For this review, take the finished solid that the model builds, in its own axes (mm). A direction names the side the tool comes from. Coordinates: 2 decimals unless noted, no trailing zeros. Write each loop counter-clockwise with the first axis right and the second up, starting at its lowest first coordinate (ties: lowest second). Pieces come first, ordered by that corner, then holes.
1) Insertion check: P1, Ø1.5, axis at x = 1, z = 23, coming from the -Y side; P2, Ø0.6, axis at x = 1.5, y = 0, coming from the -Z side. Each pin has a flat end and moves straight along its axis. Give the tip position at first contact, or say it passes through.
2) For faces 1 (the face through (0, 0, 26.6)), 2 (the face through (1, 0, -4)), list the 3-axis set-ups (+Z, -Z, +X, -X, +Y, -Y) from which the entire face can be reached by the end or side of a thin tool; tool diameter is ignored.
3) We need section A-A on z = -3. Write out the cut boundary in (x, y), then the cut area to 3 significant figures.
4) We need section B-B on z = 23.5. Write out the cut boundary in (x, y), then the cut area to 3 significant figures.
5) To check wall thickness, follow line 1 along Z through (x, y) = (1.25, 0.55); line 2 along Y through (x, z) = (0.1, -2); line 3 along Y through (x, z) = (-1, 15). State the ranges of each line that lie inside material, in increasing order.
from build123d import *

# Parameters (mm, degrees)
SKETCH_1_R           = 1.5
EXTRUDE_1_DEPTH      = 26.6
SKETCH_2_R           = 1.5
EXTRUDE_2_DEPTH      = 8.67
CHAMFER_1_SIZE       = 0.1
SKETCH_3_OUTSIDE_W   = 12.104
SKETCH_3_OUTSIDE_H   = 12.104
SKETCH_3_OUTSIDE_W_2 = 2.5
SKETCH_3_OUTSIDE_H_2 = 3
CUT_EXTRUDE_1_DEPTH  = 8.67


with BuildPart() as part:
    # Эскиз1 → Бобышка-Вытянуть1 (new body)
    with BuildSketch(Plane.XY):
        Circle(SKETCH_1_R)
    extrude(amount=EXTRUDE_1_DEPTH)

    # Эскиз2 → Бобышка-Вытянуть2 (add)
    with BuildSketch(Plane(origin=(0, 0, 0), x_dir=(-1, 0, 0), z_dir=(0, 0, -1))):
        Circle(SKETCH_2_R)
    extrude(amount=EXTRUDE_2_DEPTH)

    # Фаска1
    chamfer_1_edges = [part.edges().sort_by_distance(p)[0] for p in [
        (1.5, 0, -8.67),
    ]]
    chamfer(chamfer_1_edges, length=CHAMFER_1_SIZE)

    # Эскиз3 outside → Вырез-Вытянуть1 (cut)
    with BuildSketch(Plane(origin=(0, 0, -8.67), x_dir=(-1, 0, 0), z_dir=(0, 0, -1))):
        Rectangle(SKETCH_3_OUTSIDE_W, SKETCH_3_OUTSIDE_H)
        with Locations((0.25, 0)):
            Rectangle(SKETCH_3_OUTSIDE_W_2, SKETCH_3_OUTSIDE_H_2, mode=Mode.SUBTRACT)
    extrude(amount=-CUT_EXTRUDE_1_DEPTH, mode=Mode.SUBTRACT)


solid = part.part
Result:
1. P1: stops at y = -1.48
1. P2: stops at z = 0
2. face 1: +Z, +X, -X, +Y, -Y
2. face 2: -Z, +X, +Y, -Y
3. outline: (1, -1.12) - (1, 1.12) arc R1.5 ccw (long way) to start
3. area: 6.29 mm2
4. outline: circle Ø3 at (0, 0)
4. area: 7.07 mm2
5. line 1: z = 0 to 26.6
5. line 2: y = -1.5 to 1.5
5. line 3: y = -1.12 to 1.12
